Model file for the job. Use its own axes, mm. Round coordinates to 2 decimals unless told otherwise and drop trailing zeros. Loops run counter-clockwise (first coordinate to the right, second up) from the corner with the lowest first, then second, coordinate; pieces in that order, holes last. Notation, with made-up numbers: (-34.5, -28.75) - (23.5, -28.75) arc R20 cw to (23.5, -3.75) - close; hole circle Ø3 at (27, 14.25). An arc over 180 degrees is marked (long way). Use one line per item in the form item = value.
from build123d import *

# Parameters (mm, degrees)
SKETCH1_R           = 65
SKETCH1_R_2         = 3.95
SKETCH1_R_3         = 2.4
SKETCH1_R_4         = 4
SKETCH1_R_5         = 1.475
SKETCH1_R_6         = 1.975
SKETCH1_W           = 13
SKETCH1_H           = 5
BOSS_EXTRUDE1_DEPTH = 5


with BuildPart() as part:
    # Sketch1 → Boss-Extrude1 (new body)
    with BuildSketch(Plane.XY):
        Circle(SKETCH1_R)
        Circle(SKETCH1_R_2, mode=Mode.SUBTRACT)
        with Locations((0, 52)):
            Circle(SKETCH1_R_3, mode=Mode.SUBTRACT)
        with Locations((-30, 0)):
            Circle(SKETCH1_R_3, mode=Mode.SUBTRACT)
        with Locations((0, -52)):
            Circle(SKETCH1_R_3, mode=Mode.SUBTRACT)
        with Locations((30, 0)):
            Circle(SKETCH1_R_3, mode=Mode.SUBTRACT)
        with Locations((-41.365746699, 41.365746699)):
            Circle(SKETCH1_R_4, mode=Mode.SUBTRACT)
        with Locations((-29.25, 50.662486121)):
            Circle(SKETCH1_R_4, mode=Mode.SUBTRACT)
        with Locations((-50.662486121, 29.25)):
            Circle(SKETCH1_R_4, mode=Mode.SUBTRACT)
        with Locations((50.662486121, 29.25)):
            Circle(SKETCH1_R_4, mode=Mode.SUBTRACT)
        with Locations((41.365746699, 41.365746699)):
            Circle(SKETCH1_R_4, mode=Mode.SUBTRACT)
        with Locations((29.25, 50.662486121)):
            Circle(SKETCH1_R_4, mode=Mode.SUBTRACT)
        with Locations((50.662486121, -29.25)):
            Circle(SKETCH1_R_4, mode=Mode.SUBTRACT)
        with Locations((41.365746699, -41.365746699)):
            Circle(SKETCH1_R_4, mode=Mode.SUBTRACT)
        with Locations((29.25, -50.662486121)):
            Circle(SKETCH1_R_4, mode=Mode.SUBTRACT)
        with Locations((-29.25, -50.662486121)):
            Circle(SKETCH1_R_4, mode=Mode.SUBTRACT)
        with Locations((-41.365746699, -41.365746699)):
            Circle(SKETCH1_R_4, mode=Mode.SUBTRACT)
        with Locations((-50.662486121, -29.25)):
            Circle(SKETCH1_R_4, mode=Mode.SUBTRACT)
        with Locations((-40, 10)):
            Circle(SKETCH1_R_5, mode=Mode.SUBTRACT)
        with Locations((-50, 10)):
            Circle(SKETCH1_R_5, mode=Mode.SUBTRACT)
        with Locations((-40, -10)):
            Circle(SKETCH1_R_5, mode=Mode.SUBTRACT)
        with Locations((-50, -10)):
            Circle(SKETCH1_R_5, mode=Mode.SUBTRACT)
        with Locations((50, -10)):
            Circle(SKETCH1_R_5, mode=Mode.SUBTRACT)
        with Locations((40, -10)):
            Circle(SKETCH1_R_5, mode=Mode.SUBTRACT)
        with Locations((40, 10)):
            Circle(SKETCH1_R_5, mode=Mode.SUBTRACT)
        with Locations((50, 10)):
            Circle(SKETCH1_R_5, mode=Mode.SUBTRACT)
        with Locations((-8.485281374, 8.485281374)):
            Circle(SKETCH1_R_6, mode=Mode.SUBTRACT)
        with Locations((8.485281374, 8.485281374)):
            Circle(SKETCH1_R_6, mode=Mode.SUBTRACT)
        with Locations((8.485281374, -8.485281374)):
            Circle(SKETCH1_R_6, mode=Mode.SUBTRACT)
        with Locations((-8.485281374, -8.485281374)):
            Circle(SKETCH1_R_6, mode=Mode.SUBTRACT)
        with Locations((11.5, 22.5)):
            Rectangle(SKETCH1_W, SKETCH1_H, mode=Mode.SUBTRACT)
        with Locations((-11.5, 22.5)):
            Rectangle(SKETCH1_W, SKETCH1_H, mode=Mode.SUBTRACT)
        with Locations((11.5, -22.5)):
            Rectangle(SKETCH1_W, SKETCH1_H, mode=Mode.SUBTRACT)
        with Locations((-11.5, -22.5)):
            Rectangle(SKETCH1_W, SKETCH1_H, mode=Mode.SUBTRACT)
    extrude(amount=BOSS_EXTRUDE1_DEPTH)


solid = part.part
1. Wall check: probe 1 along Y at (x, z) = (0, 1.45); probe 2 along Y at (x, z) = (-1, 1.05); probe 3 along Y at (x, z) = (44, 3.1). Give the ranges that are in metal, low to high.
Geometry check:
probe_1 = -65 to -54.4, -49.6 to -3.95, 3.95 to 49.6, 54.4 to 65
probe_2 = -64.99 to -54.18, -49.82 to -3.82, 3.82 to 49.82, 54.18 to 64.99
probe_3 = -47.84 to -44.38, -38.36 to 38.36, 44.38 to 47.84
2. Pull direction X, two halves, no side cores. Call faces 1 (the cylindrical face through (6.512, 8.572, 2.465)), 2 (the cylindrical face through (-46.847, -28.049, 2.465)), 3 (the cylindrical face through (62, 19.52, 2.46)), 4 (the flat face through (14, 1, 5)): +X half, -X half, draft (parallel to the pull), parting line (faces both ways), or undercut.
Geometry check:
face_1 = undercut
face_2 = undercut
face_3 = parting line
face_4 = draft
3. Flat gauge pins, fed straight in: pin 1 (1.5 mm diameter, centred on x = 11.5, z = 3.5, fed in from +Y); pin 2 (1 mm diameter, centred on y = 2, z = 4, fed in from -X); pin 3 (1 mm diameter, centred on x = -23.5, z = 3, fed in from +Y); pin 4 (9 mm diameter, centred on x = 41.37, y = -41.37, fed in from -Z). Where does each tip first touch, or does it go through?
Geometry check:
pin_1 = 64.1
pin_2 = -64.98
pin_3 = 60.79
pin_4 = 0
4. Cut at D-D, the plane y = 39. Give the cut face in (x, z).
Geometry check:
outline = (-52, 0) - (-44.59, 0) - (-44.59, 5) - (-52, 5) - close; (-38.14, 0) - (38.14, 0) - (38.14, 5) - (-38.14, 5) - close; (44.59, 0) - (52, 0) - (52, 5) - (44.59, 5) - close
5. Cut at A-A, the plane y = 0. Give the cut face in (x, z).
Geometry check:
outline = (-65, 0) - (-32.4, 0) - (-32.4, 5) - (-65, 5) - close; (-27.6, 0) - (-3.95, 0) - (-3.95, 5) - (-27.6, 5) - close; (3.95, 0) - (27.6, 0) - (27.6, 5) - (3.95, 5) - close; (32.4, 0) - (65, 0) - (65, 5) - (32.4, 5) - close
6. Cut at B-B, the plane x = -40. Give the cut face in (y, z) (3 decimals), plus the area to 3 significant figures.
Geometry check:
outline = (-51.235, 0) - (-45.125, 0) - (-45.125, 5) - (-51.235, 5) - close; (-37.606, 0) - (-11.475, 0) - (-11.475, 5) - (-37.606, 5) - close; (-8.525, 0) - (8.525, 0) - (8.525, 5) - (-8.525, 5) - close; (11.475, 0) - (37.606, 0) - (37.606, 5) - (11.475, 5) - close; (45.125, 0) - (51.235, 0) - (51.235, 5) - (45.125, 5) - close
area = 408 mm^2
7. Cut at C-C, the plane x = 29.25. Give the cut face in (y, z), plus the area to 3 significant figures.
Geometry check:
outline = (-58.05, 0) - (-54.66, 0) - (-54.66, 5) - (-58.05, 5) - close; (-46.66, 0) - (-2.28, 0) - (-2.28, 5) - (-46.66, 5) - close; (2.28, 0) - (46.66, 0) - (46.66, 5) - (2.28, 5) - close; (54.66, 0) - (58.05, 0) - (58.05, 5) - (54.66, 5) - close
area = 478 mm^2
